Verification items for the finished model (mm, model axes). A direction names the side the tool comes from. Round coordinates to 2 decimals unless told otherwise and drop trailing zeros. Order: outer loops, then holes, each group sorted by start corner. A loop starts at its lowest first (then second) coordinate and runs counter-clockwise, first axis right, second up. Notation, with made-up numbers: (-2.5, 47) -> (23.5, 47) arc R9 ccw to (23.5, 62) -> close; hole circle Ø7 at (34, -1.5). An arc over 180 degrees is marked (long way). Put each result on its own line as item: value.
from build123d import *

# Parameters (mm, degrees)
F0_R     = 2.413
F0_R_2   = 1.375
F1_DEPTH = 6.35


with BuildPart() as f1:
    # F0 (on Top) → F1 (new body)
    with BuildSketch(Plane.XY):
        with BuildLine():
            ThreePointArc((-72.523684, -45.244084), (-70.663812, -49.734212), (-66.173684, -51.594084))
            Line((-66.173684, -51.594084), (73.526316, -51.594084))
            ThreePointArc((73.526316, -51.594084), (78.016444, -49.734212), (79.876316, -45.244084))
            Line((79.876316, -45.244084), (79.876316, 43.655916))
            ThreePointArc((79.876316, 43.655916), (78.016444, 48.146044), (73.526316, 50.005916))
            Line((73.526316, 50.005916), (-66.173684, 50.005916))
            ThreePointArc((-66.173684, 50.005916), (-70.663812, 48.146044), (-72.523684, 43.655916))
            Line((-72.523684, 43.655916), (-72.523684, -45.244084))
        make_face()
        with Locations((-66.173684, -45.244084)):
            Circle(F0_R, mode=Mode.SUBTRACT)
        with Locations((-29, -24.5)):
            Circle(F0_R_2, mode=Mode.SUBTRACT)
        with Locations((73.526316, -45.244084)):
            Circle(F0_R, mode=Mode.SUBTRACT)
        with Locations((29, -24.5)):
            Circle(F0_R_2, mode=Mode.SUBTRACT)
        with BuildLine():
            ThreePointArc((-32.5, 19.4125), (-32.035032, 20.535032), (-30.9125, 21))
            Line((-30.9125, 21), (-28.175, 21))
            ThreePointArc((-28.175, 21), (-25.929936, 21.929936), (-25, 24.175))
            Line((-25, 24.175), (-25, 25.4125))
            ThreePointArc((-25, 25.4125), (-24.535032, 26.535032), (-23.4125, 27))
            Line((-23.4125, 27), (23.4125, 27))
            ThreePointArc((23.4125, 27), (24.535032, 26.535032), (25, 25.4125))
            Line((25, 25.4125), (25, 24.175))
            ThreePointArc((25, 24.175), (25.929936, 21.929936), (28.175, 21))
            Line((28.175, 21), (30.9125, 21))
            ThreePointArc((30.9125, 21), (32.035032, 20.535032), (32.5, 19.4125))
            Line((32.5, 19.4125), (32.5, -19.4125))
            ThreePointArc((32.5, -19.4125), (32.035032, -20.535032), (30.9125, -21))
            Line((30.9125, -21), (28.175, -21))
            ThreePointArc((28.175, -21), (25.929936, -21.929936), (25, -24.175))
            Line((25, -24.175), (25, -25.4125))
            ThreePointArc((25, -25.4125), (24.535032, -26.535032), (23.4125, -27))
            Line((23.4125, -27), (-23.4125, -27))
            ThreePointArc((-23.4125, -27), (-24.535032, -26.535032), (-25, -25.4125))
            Line((-25, -25.4125), (-25, -24.175))
            ThreePointArc((-25, -24.175), (-25.929936, -21.929936), (-28.175, -21))
            Line((-28.175, -21), (-30.9125, -21))
            ThreePointArc((-30.9125, -21), (-32.035032, -20.535032), (-32.5, -19.4125))
            Line((-32.5, -19.4125), (-32.5, 19.4125))
        make_face(mode=Mode.SUBTRACT)
        with Locations((-29, 24.5)):
            Circle(F0_R_2, mode=Mode.SUBTRACT)
        with Locations((-66.173684, 43.655916)):
            Circle(F0_R, mode=Mode.SUBTRACT)
        with Locations((29, 24.5)):
            Circle(F0_R_2, mode=Mode.SUBTRACT)
        with Locations((73.526316, 43.655916)):
            Circle(F0_R, mode=Mode.SUBTRACT)
    extrude(amount=F1_DEPTH)


solid = f1.part
Item 1: Section check C-C on z = 4.5. State how many separate pieces and enclosed holes the cut face has, then the cut area to 3 significant figures.
Check sheet entries:
separate pieces: 1
enclosed holes: 9
area: 12,000 mm^2
Item 2: Section check A-A on y = -13.5. Record the boundary of the cut face in (x, z).
Check sheet entries:
outline: (-72.52, 0) -> (-32.5, 0) -> (-32.5, 6.35) -> (-72.52, 6.35) -> close; (32.5, 0) -> (79.88, 0) -> (79.88, 6.35) -> (32.5, 6.35) -> close
Item 3: Release check for a two-part mould opening along X. For faces 1 (the cylindrical face through (25.91, 21.95, 3.13)), 2 (the cylindrical face through (77.97, -49.78, 3.13)), 3 (the cylindrical face through (-63.87, 44.38, 3.13)), 4 (the flat face through (36, 0, 0)) record: +X half, -X half, draft (parallel to the pull), parting line (faces both ways), or undercut.
Check sheet entries:
face 1: undercut
face 2: +X half
face 3: undercut
face 4: draft
Item 4: Tool access check on faces 5 (the flat face through (3, -51.594, 3)), 6 (the flat face through (0, 27, 3)). Record the directions out of +Z, -Z, +X, -X, +Y, -Y that give a thin tool (end or side, any length) a straight path to the whole face; none if there is none.
Check sheet entries:
face 5: +Z, -Z, +X, -X, -Y
face 6: +Z, -Z
Item 5: Section check B-B on x = -3. Record the boundary of the cut face in (y, z), then the cut area to 3 significant figures.
Check sheet entries:
outline: (-51.59, 0) -> (-27, 0) -> (-27, 6.35) -> (-51.59, 6.35) -> close; (27, 0) -> (50.01, 0) -> (50.01, 6.35) -> (27, 6.35) -> close
area: 302 mm^2
Item 6: Material ranges on L1, parallel to Y at x = 29, z = 4 (3 decimals); L2, parallel to Y at x = -2.5, z = 4.5; L3, parallel to X at y = -12, z = 1.5, recorded low to high. Write a range as [from, to].
Check sheet entries:
L1: y = [-51.594, -25.875], [-23.125, -21], [21, 23.125], [25.875, 50.006]
L2: y = [-51.59, -27], [27, 50.01]
L3: x = [-72.52, -32.5], [32.5, 79.88]
